Check sheet for the drawn part. Datum: minimum x, y, z corner. Units: mm. A direction names the side the tool comes from. Round coordinates to 2 decimals unless told otherwise and drop trailing zeros. Write each loop counter-clockwise with the first axis right and the second up, starting at its lowest first coordinate (ties: lowest second). Pieces come first, ordered by that corner, then holes. Notation, with made-up numbers: M 41,7 L 73,7 A14 ccw 73,23 Z; hole C -4,44 d1. An arc over 180 degrees is marked long. Use a Markdown table: item, result.
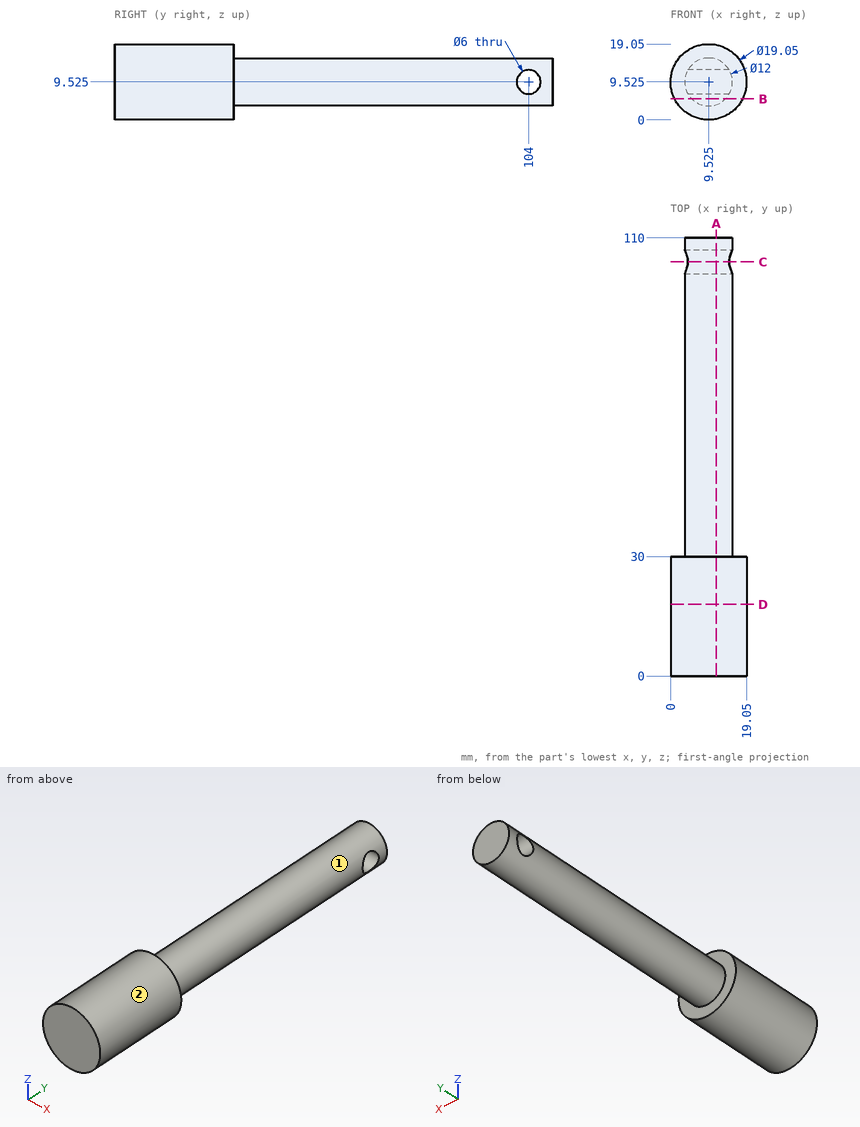
Item 1: Cross-section at A-A, the plane x = 11.5. Record the cut outline in (y, z) (3 decimals).
Outcome:
| item | result |
|---|---|
| outline | M 0,0.207 L 30,0.207 L 30,3.859 L 110,3.859 L 110,15.191 L 30,15.191 L 30,18.843 L 0,18.843 Z; hole C 104,9.525 d6 |
Item 2: Material ranges on line 1 along Z through (x, y) = (7.5, 104) (3 decimals); line 2 along Y through (x, z) = (14.25, 3.5); line 3 along X through (y, z) = (38.5, 10), recorded low to high. Write a range as from..to.
Outcome:
| item | result |
|---|---|
| line 1 | z = 3.877..6.525, 12.525..15.173 |
| line 2 | y = 0..30 |
| line 3 | x = 3.54..15.51 |
Item 3: Cross-section at D-D, the plane y = 18. Record the cut outline in (x, z) (3 decimals), and give its area (3 significant figures).
Outcome:
| item | result |
|---|---|
| outline | C 9.525,9.525 d19.05 |
| area | 285 mm2 |
Item 4: Cross-section at B-B, the plane z = 5.25. Record the cut outline in (x, y).
Outcome:
| item | result |
|---|---|
| outline | M 1.01,0 L 18.04,0 L 18.04,30 L 13.74,30 L 13.74,110 L 5.31,110 L 5.31,30 L 1.01,30 Z |
Item 5: Access from +Z, -Z, +X, -X, +Y, -Y to the whole of each face (thin tool, end or side, straight path). Record for the marked faces 1 and 2.
Outcome:
| item | result |
|---|---|
| face 1 | +Y |
| face 2 | +Y, -Y |
Item 6: Go/stop test with flat-tipped pins: pin 1 (5 mm diameter, centred on y = 104, z = 9.525, fed in from +X); pin 2 (4 mm diameter, centred on y = 91, z = 11.5, fed in from -X) (3 decimals); pin 3 (10 mm diameter, centred on x = 5.5, y = 66, fed in from +Z) (3 decimals); pin 4 (8 mm diameter, centred on y = 78, z = 7.5, fed in from +X) (3 decimals). Record where each tip stops, or that it passes through.
Outcome:
| item | result |
|---|---|
| pin 1 | passes through |
| pin 2 | stops at x = 3.525 |
| pin 3 | stops at z = 15.525 |
| pin 4 | stops at x = 15.525 |
Item 7: Cross-section at C-C, the plane y = 104. Record the cut outline in (x, z) (3 decimals), and give its area (3 significant figures).
Outcome:
| item | result |
|---|---|
| outline | M 4.329,6.525 A6 ccw 14.721,6.525 Z; M 4.329,12.525 L 14.721,12.525 A6 ccw Z |
| area | 44.2 mm2 |
